Verification items for the finished model (mm, model axes). A direction names the side the tool comes from. Coordinates: 2 decimals unless noted, no trailing zeros. Loops run counter-clockwise (first coordinate to the right, second up) from the corner with the lowest first, then second, coordinate; pieces in that order, holes last. Notation, with made-up numbers: (73, 24) - (89, 24) arc R24 ccw to (89, 53) - close; hole circle Ø10 at (83.25, 34). An arc over 180 degrees is marked (long way). One line per item, written item: value. Start each with the question number.
(1) Set-up check for faces 1 (the face through (423.846, 7.509, 49.65)), 2 (the face through (-185, 1, 50)), 3 (the face through (449.99, 1.07, -11.98)): record each of +Z, -Z, +X, -X, +Y, -Y from which the full face is reachable in a straight line by a thin tool's end or side.
(2) Thickness scan on probe 1 along X at (y, z) = (0, -9); probe 2 along Y at (x, z) = (-290, -12); probe 3 along Z at (x, y) = (-65, 33). Record the ranges inside material, lowest first. Write a range as [from, to].
(3) Section check B-B (x = 283). Record the boundary of the cut face in (y, z).
(4) Draft check along Y on faces 4 (the face through (138.65, 59.51, 6.96)), 5 (the face through (-339.95, 2.2, 0.7)), 6 (the face through (48, 1, -50)). Enter one of: +Y half, -Y half, draft (parallel to the pull), parting line (faces both ways), or undercut.
(5) Section check C-C (z = 101). Record the boundary of the cut face in (x, y).
(6) Gauge pin test, flat ends, axial feed: P1, Ø1.5, axis at x = -173, y = 27.5, coming from the +Z side; P2, Ø5, axis at x = 275, y = -19, coming from the +Z side; P3, Ø1.5, axis at y = 27.5, z = 121, coming from the -X side. Record the tip position at first contact, or that the pin passes through.
(7) Section check A-A (y = 0). Record the boundary of the cut face in (x, z), plus the area to 3 significant figures.
```python
from build123d import *
from build123d.topology import SkipClean

# Parameters (mm, degrees)
SKETCH2_R                      = 50
BOSS_EXTRUDE1_DEPTH            = 50
BOSS_EXTRUDE4_START            = 100
SKETCH6_R                      = 50
BOSS_EXTRUDE4_DEPTH            = 100
CUT_EXTRUDE1_DEPTH             = 25
CUT_EXTRUDE1_DEPTH_BACK        = 25
CUT_EXTRUDE1_START             = 50
SKETCH8_R                      = 100
SKETCH8_R_2                    = 25
CUT_EXTRUDE2_REACH             = 482.234
CUT_EXTRUDE2_DIRECTION_2_REACH = 482.234
FILLET1_R                      = 200


with BuildPart() as part:
    # Sketch2 → Boss-Extrude1 (new, symmetric)
    with BuildSketch(Plane.XY):
        with BuildLine():
            Line((-287.282608696, 74.95075573), (401.811594203, 49.967170487))
            ThreePointArc((401.811594203, 49.967170487), (450, 0), (401.811594203, -49.967170487))
            Line((401.811594203, -49.967170487), (-287.282608696, -74.95075573))
            ThreePointArc((-287.282608696, -74.95075573), (-365, 0), (-287.282608696, 74.95075573))
        make_face()
        with Locations((-290, 0)):
            Circle(SKETCH2_R, mode=Mode.SUBTRACT)
    extrude(amount=BOSS_EXTRUDE1_DEPTH, both=True)

    # Sketch6 → Boss-Extrude4 (add)
    with SkipClean():  # the faces are left unmerged after this step: merging them gives an invalid solid
        with BuildSketch(Plane.XY.offset(50).offset(BOSS_EXTRUDE4_START)):
            with BuildLine():
                Line((-287.282608696, -74.95075573), (401.811594203, -49.967170487))
                ThreePointArc((401.811594203, -49.967170487), (450, 0), (401.811594203, 49.967170487))
                Line((401.811594203, 49.967170487), (-287.282608696, 74.95075573))
                ThreePointArc((-287.282608696, 74.95075573), (-365, 0), (-287.282608696, -74.95075573))
            make_face()
            with Locations((-290, 0)):
                Circle(SKETCH6_R, mode=Mode.SUBTRACT)
        extrude(amount=-BOSS_EXTRUDE4_DEPTH)

    # Sketch8 → Cut-Extrude1 (cut, two sides: drawn at the far end of the back side and taken through both)
    with SkipClean():  # the faces are left unmerged after this step: merging them gives an invalid solid
        with BuildSketch(Plane.XY.offset(CUT_EXTRUDE1_START - CUT_EXTRUDE1_DEPTH_BACK)):
            with Locations((400, 0)):
                Circle(SKETCH8_R)
            with Locations((400, 0)):
                Circle(SKETCH8_R_2, mode=Mode.SUBTRACT)
        extrude(amount=CUT_EXTRUDE1_DEPTH + CUT_EXTRUDE1_DEPTH_BACK, mode=Mode.SUBTRACT)

    # Sketch9 → Cut-Extrude2 (cut, up to next)
    with BuildSketch(Plane(origin=(0, 0, 0), x_dir=(1, 0, 0), z_dir=(0, 1, 0)), mode=Mode.PRIVATE) as cut_extrude2_sk1:
        with BuildLine():
            Line((-365, -50), (0, -50))
            ThreePointArc((0, -50), (158.113883008, -75.658350975), (300, -150))
            Line((300, -150), (-365, -150))
            Line((-365, -150), (-365, -50))
        make_face()
    cut_extrude2_tool1 = extrude(cut_extrude2_sk1.sketch, amount=-CUT_EXTRUDE2_REACH, mode=Mode.PRIVATE) & part.part
    add(cut_extrude2_tool1.solids().sort_by_distance((-76.011524, 0, 103.458826))[0], mode=Mode.SUBTRACT)

    # Sketch9 → Cut-Extrude2 direction 2 (cut, up to next)
    with BuildSketch(Plane(origin=(0, 0, 0), x_dir=(1, 0, 0), z_dir=(0, 1, 0)), mode=Mode.PRIVATE) as cut_extrude2_direction_2_sk1:
        with BuildLine():
            Line((-365, -50), (0, -50))
            ThreePointArc((0, -50), (158.113883008, -75.658350975), (300, -150))
            Line((300, -150), (-365, -150))
            Line((-365, -150), (-365, -50))
        make_face()
    cut_extrude2_direction_2_tool1 = extrude(cut_extrude2_direction_2_sk1.sketch, amount=CUT_EXTRUDE2_DIRECTION_2_REACH, mode=Mode.PRIVATE) & part.part
    add(cut_extrude2_direction_2_tool1.solids().sort_by_distance((-76.011524, 0, 103.458826))[0], mode=Mode.SUBTRACT)

    # Fillet1
    fillet1_edges = [part.edges().sort_by_distance(p)[0] for p in [
        (300, 0, 150),
    ]]
    fillet(fillet1_edges, radius=FILLET1_R)


solid = part.part
```
Responses:
1. face 1: none
1. face 2: +Z, -X, +Y, -Y
1. face 3: +Z, -Z, +X
2. probe 1: x = [-365, -340], [-240, 450]
2. probe 2: y = [-75, -50], [50, 75]
2. probe 3: z = [-50, 50]
3. outline: (-54.27, -50) - (54.27, -50) - (54.27, 134.35) - (-54.27, 134.35) - close
4. face 4: +Y half
4. face 5: undercut
4. face 6: draft
5. outline: (220, -56.56) - (401.81, -49.97) arc R50 ccw to (401.81, 49.97) - (220, 56.56) - close
6. P1: stops at z = 50
6. P2: stops at z = 131.94
6. P3: stops at x = 255.57
7. outline: (-365, -50) - (-340, -50) - (-340, 50) - (-365, 50) - close; (-240, -50) - (450, -50) - (450, 25) - (425, 25) - (425, 75) - (450, 75) - (450, 150) - (360.56, 150) arc R200 ccw to (257.54, 121.43) arc R500 cw to (0, 50) - (-240, 50) - close; hole (300, 25) - (375, 25) - (375, 75) - (300, 75) - close
7. area: 90,700 mm²
